The figure shows three views and two pictorial views of one solid part (mm, origin at its lowest corner). Answer the questions. A direction names the side the tool comes from. Coordinates: 2 decimals unless noted, no trailing zeros. Loops run counter-clockwise (first coordinate to the right, second up) from the corner with the lowest first, then second, coordinate; pieces in that order, holes last. Notation, with made-up numbers: M 38,-16.75 L 54,-16.75 A10 cw 54,-8.75 Z; hole C 37.5,-20.5 d1. An arc over 180 degrees is marked long. Write each question's results on one line, items separated by ' | '.
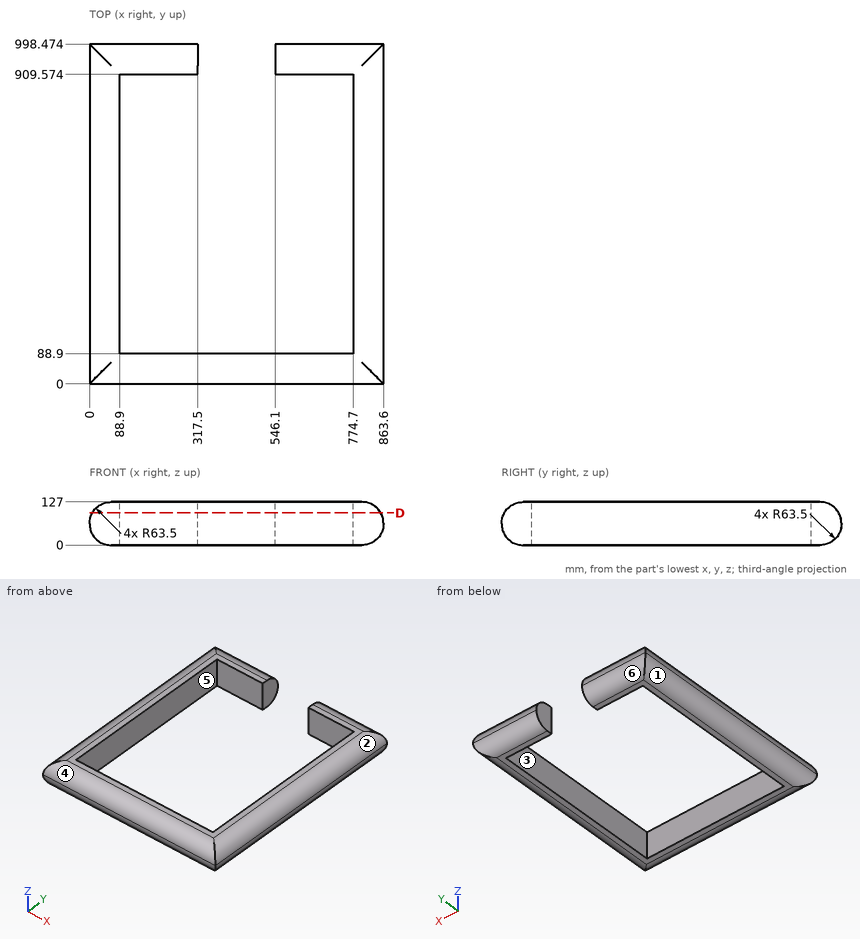
1) Given pin 1 Ø3 at (y, z) = (577, 95.5) entering from -X; pin 2 Ø4 at (x, z) = (673, 25.5) entering from -Y; pin 3 Ø1 at (x, z) = (429, 97.5) entering from -Y, each flat-ended and moving along its own axis, determine where each tip first touches the part or whether it passes through.
Check result:
pin 1: x = 7.8 | pin 2: y = 11.19 | pin 3: y = 9.56
2) Which of the six approach directions +Z, -Z, +X, -X, +Y, -Y give full straight-line access (tool end or side, diameter ignored) to the marked faces 5 and 6?
Check result:
face 5: +Z, -Z | face 6: -Z, +X, -X, +Y
3) Find section D-D, the plane z = 95. Give the vertices of the cut face in (x, y).
Check result:
outline: M 8.36,8.36 L 855.24,8.36 L 855.24,990.11 L 546.1,990.11 L 546.1,909.57 L 774.7,909.57 L 774.7,88.9 L 88.9,88.9 L 88.9,909.57 L 317.5,909.57 L 317.5,990.11 L 8.36,990.11 Z
4) For a pull along X with two mould halves and no side action, classify the marked faces 1, 2, 3 and 4 as released by +X, released by -X, zero draft, split by the parting line, or undercut.
Check result:
face 1: released by -X | face 2: released by +X | face 3: undercut | face 4: zero draft
5) Straight lines are drawn through the part: probe 1 along X at (y, z) = (847, 66); probe 2 along Y at (x, z) = (210, 60); probe 3 along Y at (x, z) = (104, 10.5) (1 decimal). For each, find the intervals that lie inside material, in ascending order. Write a range as [from, to].
Check result:
probe 1: [0.05, 88.9], [774.7, 863.55] | probe 2: [0.1, 88.9], [909.57, 998.38] | probe 3: [28.5, 88.9], [909.6, 969.9]
